For this review, take the finished solid that the model builds, in its own axes (mm). Coordinates: 2 decimals unless noted, no trailing zeros. Loops run counter-clockwise (first coordinate to the right, second up) from the corner with the lowest first, then second, coordinate; pieces in that order, holes last. Notation, with made-up numbers: (6.25, -31.75) - (57.25, -31.75) arc R16 ccw to (57.25, -18.75) - close; hole circle Ø10 at (60, 82.5). An arc over 180 degrees is marked (long way). Use one line per item in the form item = value. Start each with the question number.
1. Add section C-C on z = -3.5. Give the boundary of the cut face in (x, y) (1 decimal).
2. Draft analysis for pull direction X (two halves, no side actions). For faces 1 (the face through (11.9, 0.2, -0.1)), 2 (the face through (-17.462, 0, 0)), 3 (the face through (0, 9.525, 0)), state which applies: +X half, -X half, draft (parallel to the pull), parting line (faces both ways), or undercut.
3. Add section B-B on x = 7. Give the boundary of the cut face in (y, z) (1 decimal), and give its area (3 significant figures).
4. Add section A-A on y = 0. Give the boundary of the cut face in (x, z).
5. To check wall thickness, follow probe 1 along X at (y, z) = (-1.25, -2); probe 2 along X at (y, z) = (-1.5, 1.25); probe 3 along X at (y, z) = (-2.5, -3). State the ranges of each line that lie inside material, in increasing order.
6. Add section D-D on y = 3.5. Give the boundary of the cut face in (x, z).
7. For pin 1 Ø5 at (x, y) = (7.94, 0) entering from +Z, flat-tipped, find the tip position at first contact; note if it passes through.
```python
from build123d import *

# Parameters (mm, degrees)
F0_W     = 19.05
F0_H     = 9.525
F1_DEPTH = 17.4625
F3_D     = 7.9375
F5_D     = 3.4544


with BuildPart() as f1:
    # F0 (on Right) → F1 (new body, symmetric)
    with BuildSketch(Plane.YZ):
        Rectangle(F0_W, F0_H)
    extrude(amount=F1_DEPTH, both=True)

    # F3 (through all)
    with Locations(Plane.XY.offset(4.7625)):
        with Locations((7.9375, 0)):
            Hole(F3_D / 2)

    # F5 (through all)
    with Locations(Plane.XY.offset(4.7625)):
        with Locations((-11.1125, 0)):
            Hole(F5_D / 2)


solid = f1.part
```
Conclusion:
q1.outline = (-17.5, -9.5) - (17.5, -9.5) - (17.5, 9.5) - (-17.5, 9.5) - close; hole circle Ø3.5 at (-11.1, 0); hole circle Ø7.9 at (7.9, 0)
q2.face_1 = undercut
q2.face_2 = -X half
q2.face_3 = draft
q3.outline = (-9.5, -4.8) - (-3.9, -4.8) - (-3.9, 4.8) - (-9.5, 4.8) - close; (3.9, -4.8) - (9.5, -4.8) - (9.5, 4.8) - (3.9, 4.8) - close
q3.area = 108 mm^2
q4.outline = (-17.46, -4.76) - (-12.84, -4.76) - (-12.84, 4.76) - (-17.46, 4.76) - close; (-9.39, -4.76) - (3.97, -4.76) - (3.97, 4.76) - (-9.39, 4.76) - close; (11.91, -4.76) - (17.46, -4.76) - (17.46, 4.76) - (11.91, 4.76) - close
q5.probe_1 = -17.46 to -12.3, -9.92 to 4.17, 11.7 to 17.46
q5.probe_2 = -17.46 to -11.97, -10.26 to 4.26, 11.61 to 17.46
q5.probe_3 = -17.46 to 4.86, 11.02 to 17.46
q6.outline = (-17.46, -4.76) - (6.07, -4.76) - (6.07, 4.76) - (-17.46, 4.76) - close; (9.81, -4.76) - (17.46, -4.76) - (17.46, 4.76) - (9.81, 4.76) - close
q7.pin_1 = through
